Check sheet for the modelled part. Datum: model origin and axes. Units: mm. Face numbers are marked on the shaded views. A direction names the side the tool comes from. Coordinates: 2 decimals unless noted, no trailing zeros. Loops run counter-clockwise (first coordinate to the right, second up) from the corner with the lowest first, then second, coordinate; pieces in that order, holes last.
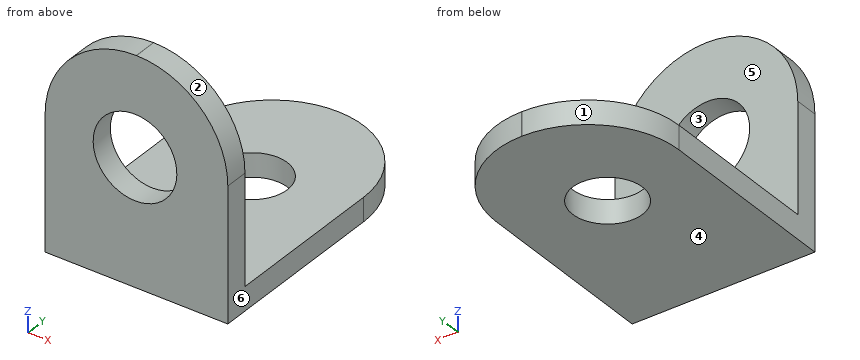
```python
from build123d import *

# Parameters (mm, degrees)
SKETCH1_W           = 16.1
SKETCH1_H           = 20
BOSS_EXTRUDE1_DEPTH = 13.1
SKETCH2_W           = 14.4
SKETCH2_H           = 18.3
CUT_EXTRUDE1_DEPTH  = 26.915439414
FILLET1_R           = 6.545
SKETCH20_R          = 3
CUT_EXTRUDE2_DEPTH  = 10
SKETCH21_R          = 2.5
CUT_EXTRUDE3_DEPTH  = 10


with BuildPart() as part:
    # Sketch1 → Boss-Extrude1 (new body)
    with BuildSketch(Plane(origin=(6.653968254, 0, 0), x_dir=(0, 0, -1), z_dir=(1, 0, 0))):
        with Locations((1.95, 10)):
            Rectangle(SKETCH1_W, SKETCH1_H)
    extrude(amount=-BOSS_EXTRUDE1_DEPTH)

    # Sketch2 → Cut-Extrude1 (cut, through all)
    with BuildSketch(Plane.ZY.offset(6.446031746)):
        with Locations((-1.1, 10.85)):
            Rectangle(SKETCH2_W, SKETCH2_H)
    extrude(amount=-CUT_EXTRUDE1_DEPTH, mode=Mode.SUBTRACT)

    # Fillet1
    fillet1_edges = [part.edges().sort_by_distance(p)[0] for p in [
        (-6.446031746, 20, -9.15),
        (6.653968254, 0.85, 6.1),
        (-6.446031746, 0.85, 6.1),
        (6.653968254, 20, -9.15),
    ]]
    fillet(fillet1_edges, radius=FILLET1_R)

    # Sketch20 → Cut-Extrude2 (cut)
    with BuildSketch(Plane.XZ):
        with Locations(Location((0, -1, 0), (0, 0, 270))):
            Circle(SKETCH20_R)
    extrude(amount=-CUT_EXTRUDE2_DEPTH, mode=Mode.SUBTRACT)

    # Sketch21 → Cut-Extrude3 (cut)
    with BuildSketch(Plane(origin=(0, 0, -10), x_dir=(-1, 0, 0), z_dir=(0, 0, -1))):
        with Locations(Location((-0.098968254, 11.5, 0), (0, 0, 90))):
            Circle(SKETCH21_R)
    extrude(amount=-CUT_EXTRUDE3_DEPTH, mode=Mode.SUBTRACT)


solid = part.part
```
1) Set-up check for the marked faces 5 and 6: record each of +Z, -Z, +X, -X, +Y, -Y from which the full face is reachable in a straight line by a thin tool's end or side.
Answer sheet:
face 5: +Z, +X, -X, +Y
face 6: +Z, -Z, +X, +Y, -Y
2) Section check C-C on x = 0.75. Enter the section's corners in (y, z).
Answer sheet:
outline: (0, -10) - (9.09, -10) - (9.09, -8.3) - (1.7, -8.3) - (1.7, -3.9) - (0, -3.9) - close; (0, 1.9) - (1.7, 1.9) - (1.7, 6.07) - (0, 6.07) - close; (13.91, -10) - (19.97, -10) - (19.97, -8.3) - (13.91, -8.3) - close
3) Depth check by flat-ended pin: pin 1 (1.5 mm diameter, centred on x = -3.5, z = 3, fed in from +Y); pin 2 (2 mm diameter, centred on x = 4.5, y = 4.5, fed in from +Z). Enter the tip coordinate at first touch or a pass-through.
Answer sheet:
pin 1: stops at y = 1.7
pin 2: stops at z = -8.3
4) Section check A-A on y = 11.5. Enter the section's corners in (x, z), plus the area to 3 significant figures.
Answer sheet:
outline: (-6.45, -10) - (-2.4, -10) - (-2.4, -8.3) - (-6.45, -8.3) - close; (2.6, -10) - (6.65, -10) - (6.65, -8.3) - (2.6, -8.3) - close
area: 13.8 mm2
5) Mould release check, pull along Z, two halves, no side actions. Record for the marked faces 1, 2, 3 and 4: +Z half, -Z half, draft (parallel to the pull), parting line (faces both ways), or undercut.
Answer sheet:
face 1: draft
face 2: +Z half
face 3: undercut
face 4: -Z half
6) Section check B-B on z = -1. Enter the section's corners in (x, y).
Answer sheet:
outline: (-6.45, 0) - (-3, 0) - (-3, 1.7) - (-6.45, 1.7) - close; (3, 0) - (6.65, 0) - (6.65, 1.7) - (3, 1.7) - close
7) Scan lines: line 1 (Z direction, x = 6, y = 11.5); line 2 (X direction, y = 11.5, z = -9.3); line 3 (Y direction, x = 5.75, z = 1.25). Record each from-to range of solid material in increasing order.
Answer sheet:
line 1: z = -10 to -8.3
line 2: x = -6.45 to -2.4, 2.6 to 6.65
line 3: y = 0 to 1.7
8) Section check D-D on z = -6.5. Enter the section's corners in (x, y).
Answer sheet:
outline: (-6.45, 0) - (6.65, 0) - (6.65, 1.7) - (-6.45, 1.7) - close
